from build123d import *

# Parameters (mm, degrees)
SKETCH_R          = 11
PAD_DEPTH         = 2
SKETCH002_R       = 4
SKETCH002_R_2     = 1.75
POCKET_DEPTH      = 2.001
SKETCH003_R       = 5
PAD001_DEPTH      = 10
PAD001_DEPTH_BACK = 5.6
SKETCH004_R       = 4
POCKET001_DEPTH   = 15.601


with BuildPart() as part:
    # Sketch → Pad (new body)
    with BuildSketch(Plane.XY):
        Circle(SKETCH_R)
    extrude(amount=PAD_DEPTH)

    # Sketch002 (on Face3 of Pad) → Pocket (cut, through all)
    with BuildSketch(Plane.XY.offset(2)):
        Circle(SKETCH002_R)
        with Locations((0, -7.75)):
            Circle(SKETCH002_R_2)
        with Locations((-7.75, 0)):
            Circle(SKETCH002_R_2)
        with Locations((0, 7.75)):
            Circle(SKETCH002_R_2)
        with Locations((7.75, 0)):
            Circle(SKETCH002_R_2)
    extrude(amount=-POCKET_DEPTH, mode=Mode.SUBTRACT)

    # Sketch003 (on Face3 of Pocket) → Pad001 (join, two sides)
    with BuildSketch(Plane.XY.offset(2)) as pad001_sk:
        Circle(SKETCH003_R)
    extrude(amount=PAD001_DEPTH)
    extrude(pad001_sk.sketch, amount=-PAD001_DEPTH_BACK)

    # Sketch004 (on Face11 of Pad001) → Pocket001 (cut, through all)
    with BuildSketch(Plane.XY.offset(12)):
        Circle(SKETCH004_R)
    extrude(amount=-POCKET001_DEPTH, mode=Mode.SUBTRACT)


solid = part.part
Could you check a few things on this model? Use its own coordinates, in mm. A direction names the side the tool comes from. Give positions to 0.01 mm unless a question says otherwise; leave off trailing zeros. Loops run counter-clockwise (first coordinate to the right, second up) from the corner with the lowest first, then second, coordinate; pieces in that order, holes last. Notation, with made-up numbers: (-14, 29.5) -> (34, 29.5) arc R19 cw to (34, 49.5) -> close; hole circle Ø8 at (53, -7.5). An arc over 180 degrees is marked (long way). Answer as CSV lines item,"result". Start each with the question number.
(1) We'd pull the mould along Y, two halves only. Please class faces 4 (the cylindrical face through (-2.38, -10.74, 0.99)), 5 (the cylindrical face through (-0.228, 9.485, 1.014)), 6 (the flat face through (5, -2, 0)), 7 (the cylindrical face through (9.419, 0.526, 1.014)): released by +Y, released by -Y, zero draft, split by the parting line, or undercut.
(2) I'm going to push flat-ended pins straight in: pin 1 Ø4.5 at (x, y) = (0, 7.75) entering from +Z; pin 2 Ø2 at (x, z) = (-2, 7.5) entering from -Y; pin 3 Ø3 at (x, z) = (-1, 2.5) entering from +Y; pin 4 Ø4 at (x, y) = (0, -7.75) entering from -Z. Where does each tip first touch, or does it pass through?
(3) If we section it at C-C on x = -7.5: Write out the boundary of the cut face in (y, z).
(4) If we section it at D-D on y = -7.75: Write out the boundary of the cut face in (x, z), then the cut area to 3 significant figures.
(5) Which directions (+Z, -Z, +X, -X, +Y, -Y) give clear straight access to the entire face, cutting with the end or side of a thin tool? Please do faces 1 (the cylindrical face through (0.81, -9.3, 1.01)), 2 (the cylindrical face through (-1.08, -4.88, 6.93)), 3 (the cylindrical face through (-1.08, -4.88, -1.77)).
(6) I need wall thicknesses on probe 1 along Y at (x, z) = (-1, 1); probe 2 along Y at (x, z) = (0, 6); probe 3 along Z at (x, y) = (8.5, 3.5). Which ranges of each line are inside material? Lowest first, please.
(7) If we section it at A-A on y = 0: Write out the boundary of the cut face in (x, z).
Computed:
1,face 4,"split by the parting line"
1,face 5,"undercut"
1,face 6,"zero draft"
1,face 7,"undercut"
2,pin 1,"stops at z = 2"
2,pin 2,"stops at y = -4.9"
2,pin 3,"stops at y = 11"
2,pin 4,"stops at z = 0"
3,outline,"(-8.05, 0) -> (-1.73, 0) -> (-1.73, 2) -> (-8.05, 2) -> close; (1.73, 0) -> (8.05, 0) -> (8.05, 2) -> (1.73, 2) -> close"
4,outline,"(-7.81, 0) -> (-1.75, 0) -> (-1.75, 2) -> (-7.81, 2) -> close; (1.75, 0) -> (7.81, 0) -> (7.81, 2) -> (1.75, 2) -> close"
4,area,"24.2 mm2"
5,face 1,"+Z, -Z"
5,face 2,"+Z"
5,face 3,"-Z"
6,probe 1,"y = -10.95 to -9.19, -6.31 to -3.87, 3.87 to 6.31, 9.19 to 10.95"
6,probe 2,"y = -5 to -4, 4 to 5"
6,probe 3,"z = 0 to 2"
7,outline,"(-11, 0) -> (-9.5, 0) -> (-9.5, 2) -> (-11, 2) -> close; (-6, 0) -> (-5, 0) -> (-5, -3.6) -> (-4, -3.6) -> (-4, 12) -> (-5, 12) -> (-5, 2) -> (-6, 2) -> close; (4, -3.6) -> (5, -3.6) -> (5, 0) -> (6, 0) -> (6, 2) -> (5, 2) -> (5, 12) -> (4, 12) -> close; (9.5, 0) -> (11, 0) -> (11, 2) -> (9.5, 2) -> close"
